Geometry: final body of the model. Coordinates: model frame, mm. Face numbers are marked on the shaded views. A direction names the side the tool comes from. Coordinates: 2 decimals unless noted, no trailing zeros. Write each loop counter-clockwise with the first axis right and the second up, starting at its lowest first coordinate (ties: lowest second). Pieces come first, ordered by that corner, then holes.
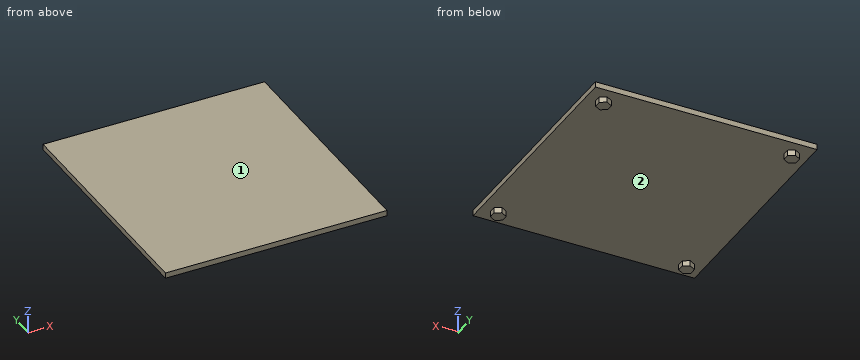
from build123d import *

# Parameters (mm, degrees)
CROQUIS1_W              = 400
CROQUIS1_H              = 426.64
SALIENTE_EXTRUIR1_DEPTH = 10
SALIENTE_EXTRUIR2_DEPTH = 10


with BuildPart() as part:
    # Croquis1 → Saliente-Extruir1 (new body)
    with BuildSketch(Plane.XY):
        Rectangle(CROQUIS1_W, CROQUIS1_H)
    extrude(amount=SALIENTE_EXTRUIR1_DEPTH)

    # Croquis2 → Saliente-Extruir2 (add)
    with BuildSketch(Plane(origin=(0, 0, 0), x_dir=(-1, 0, 0), z_dir=(0, 0, -1))):
        Polygon((-170, 170.618294078), (-159, 176.969147039), (-159, 189.670852961), (-170, 196.021705922), (-181, 189.670852961), (-181, 176.969147039), align=None)
        Polygon((-170, -170.618294078), (-181, -176.969147039), (-181, -189.670852961), (-170, -196.021705922), (-159, -189.670852961), (-159, -176.969147039), align=None)
        Polygon((170, 170.618294078), (181, 176.969147039), (181, 189.670852961), (170, 196.021705922), (159, 189.670852961), (159, 176.969147039), align=None)
        Polygon((170, -170.618294078), (159, -176.969147039), (159, -189.670852961), (170, -196.021705922), (181, -189.670852961), (181, -176.969147039), align=None)
    extrude(amount=SALIENTE_EXTRUIR2_DEPTH)


solid = part.part
Item 1: Set-up query: the marked faces 1 and 2. Return all of +Z, -Z, +X, -X, +Y, -Y with unobstructed straight access to the full face (end or side cutting, diameter ignored); none if empty.
Derived:
face 1: +Z, +X, -X, +Y, -Y
face 2: -Z
Item 2: Section B-B, the plane y = -182. Output: boundary loops of the cut face in (x, z), plus the area to 3 significant figures.
Derived:
outline: (-200, 0) - (-181, 0) - (-181, -10) - (-159, -10) - (-159, 0) - (159, 0) - (159, -10) - (181, -10) - (181, 0) - (200, 0) - (200, 10) - (-200, 10) - close
area: 4,440 mm2
Item 3: Section C-C, the plane x = 3.5. Output: boundary loops of the cut face in (y, z), plus the area to 3 significant figures.
Derived:
outline: (-213.32, 0) - (213.32, 0) - (213.32, 10) - (-213.32, 10) - close
area: 4,270 mm2
Item 4: Section D-D, the plane y = -71. Output: boundary loops of the cut face in (x, z), plus the area to 3 significant figures.
Derived:
outline: (-200, 0) - (200, 0) - (200, 10) - (-200, 10) - close
area: 4,000 mm2
Item 5: Pin query (flat end, axial travel): pin 1 (8 mm diameter, centred on y = 119, z = -3.5, fed in from -X); pin 2 (3 mm diameter, centred on y = 182, z = -4.5, fed in from -X); pin 3 (3 mm diameter, centred on y = 185.5, z = -5, fed in from +X). Return the tip coordinate at first contact, or that it passes through.
Derived:
pin 1: stops at x = -200
pin 2: stops at x = -181
pin 3: stops at x = 181
Item 6: Material intervals for probe 1 along Z at (x, y) = (107.5, 105), sorted ascending.
Derived:
probe 1: z = 0 to 10
Item 7: Section A-A, the plane z = -3.25. Output: boundary loops of the cut face in (x, y).
Derived:
outline: (-181, -189.67) - (-170, -196.02) - (-159, -189.67) - (-159, -176.97) - (-170, -170.62) - (-181, -176.97) - close; (-181, 176.97) - (-170, 170.62) - (-159, 176.97) - (-159, 189.67) - (-170, 196.02) - (-181, 189.67) - close; (159, -189.67) - (170, -196.02) - (181, -189.67) - (181, -176.97) - (170, -170.62) - (159, -176.97) - close; (159, 176.97) - (170, 170.62) - (181, 176.97) - (181, 189.67) - (170, 196.02) - (159, 189.67) - close
